from build123d import *

# Parameters (mm, degrees)
BASPROSKE_W        = 16
BASPROSKE_H        = 17
TOOTHCUT_DEPTH     = 29.879058156
TEETHCUTS_COUNT    = 15
TEETHCUTS_ANGLE    = 336
BORSKE_R           = 4
BORE_DEPTH         = 50.0000508
CUT_EXTRUDE1_DEPTH = 5


with BuildPart() as part:
    # BasProSke → Base-Revolve (revolve)
    with BuildSketch(Plane(origin=(0, 0, 0), x_dir=(1, 0, 0), z_dir=(0, 1, 0)), mode=Mode.PRIVATE) as base_revolve_sk:
        with Locations((8, 8.5)):
            Rectangle(BASPROSKE_W, BASPROSKE_H)
    revolve(base_revolve_sk.sketch.rotate(Axis((-10, 0, 0), (1, 0, 0)), 180), axis=Axis((-10, 0, 0), (1, 0, 0)))

    # TooCutSke → ToothCut (cut, through all)
    with BuildSketch(Plane(origin=(0, 0, 0), x_dir=(0, 0, -1), z_dir=(1, 0, 0))):
        with BuildLine():
            ThreePointArc((1.050056448, 12.454813626), (0, 12.499), (-1.050056448, 12.454813626))
            ThreePointArc((-1.050056448, 12.454813626), (-1.638118106, 14.809604533), (-3.110934279, 16.73876737))
            ThreePointArc((-3.110934279, 16.73876737), (0, 17.0254), (3.110934279, 16.73876737))
            ThreePointArc((3.110934279, 16.73876737), (1.638118106, 14.809604533), (1.050056448, 12.454813626))
        make_face()
    toothcut = extrude(amount=TOOTHCUT_DEPTH, mode=Mode.SUBTRACT)

    # TeethCuts: ToothCut ×15 about axis
    teethcuts_axis = Axis((-10, 0, 0), (1, 0, 0))
    for i in range(1, TEETHCUTS_COUNT):
        add(toothcut.rotate(teethcuts_axis, i * TEETHCUTS_ANGLE / (TEETHCUTS_COUNT - 1)), mode=Mode.SUBTRACT)

    # BorSke → Bore (cut, symmetric)
    with BuildSketch(Plane(origin=(0, 0, 0), x_dir=(0, 0, -1), z_dir=(1, 0, 0))):
        with Locations(Location((0, 0, 0), (0, 0, 180))):
            Circle(BORSKE_R)
    extrude(amount=BORE_DEPTH, both=True, mode=Mode.SUBTRACT)

    # Sketch1 → Cut-Extrude1 (cut)
    with BuildSketch(Plane(origin=(16, 0, 0), x_dir=(0, 0, -1), z_dir=(1, 0, 0))):
        Polygon((-3.75277675, 6.5), (-7.505553499, 0), (-3.75277675, -6.5), (3.75277675, -6.5), (7.505553499, 0), (3.75277675, 6.5), align=None)
    extrude(amount=-CUT_EXTRUDE1_DEPTH, mode=Mode.SUBTRACT)


solid = part.part
The listing builds one solid part. Answer for the finished solid, in the listing's coordinates (mm). A direction names the side the tool comes from. Round coordinates to 2 decimals unless told otherwise and drop trailing zeros. Write each loop counter-clockwise with the first axis right and the second up, starting at its lowest first coordinate (ties: lowest second). Pieces come first, ordered by that corner, then holes. Notation, with made-up numbers: (62, 43) - (99, 43) arc R37 cw to (99, 80) - close; hole circle Ø10 at (-9.5, -2). An arc over 180 degrees is marked (long way). Use one line per item in the form item = value. Start each with the question number.
Item 1: Determine the mould class of faces 4 (the cylindrical face through (7.89, -6.24, 10.83)), 5 (the flat face through (0, 3, -4)), 6 (the cylindrical face through (7.888, -14.159, 4.692)) for opening direction Y: +Y half, -Y half, draft (parallel to the pull), parting line (faces both ways), or undercut.
Item 2: A tool of negligible diameter and unlimited length cuts with its end or side. For faces 1 (the cylindrical face through (7.89, 11.41, -5.1)), 2 (the flat face through (13.54, 3.2, -5.66)), 3 (the cylindrical face through (7.9, 11.1, 9.9)), from which of +Z, -Z, +X, -X, +Y, -Y can it reach the whole face along a straight path? Write none if from no direction.
Item 3: Find the intervals of material crossed by line 1 (Y direction, x = 5, z = 0); line 2 (Y direction, x = 2.75, z = -13); line 3 (Z direction, x = 6.5, y = -10), in increasing order. Write a range as [from, to].
Item 4: A cutting plane is placed at C-C (y = -9). Write down the section's boundary in (x, z), plus the area to 3 significant figures.
Item 5: A cutting plane is placed at B-B (z = 14). Write down the section's boundary in (x, y), plus the area to 3 significant figures.
Item 6: Flat-ended cylindrical pins translate along their axes: pin 1 Ø4 at (y, z) = (1, -3) entering from +X; pin 2 Ø3 at (x, z) = (14, -12) entering from -Y; pin 3 Ø1.5 at (x, z) = (12.5, 8.5) entering from +Y. Find the tip coordinate at first contact, or state that the pin passes through.
Item 7: A cutting plane is placed at A-A (z = 0). Write down the section's boundary in (x, y).
The answers:
q1.face_4 = undercut
q1.face_5 = draft
q1.face_6 = -Y half
q2.face_1 = +X, -X
q2.face_2 = +X
q2.face_3 = +Z, +X, -X
q3.line_1 = [-17, -4], [4, 12.5]
q3.line_2 = [-5.9, -2.5], [-0.27, 3.02], [5.65, 8.88]
q3.line_3 = [-12.63, -8.65], [-7.5, 7.5], [8.65, 12.63]
q4.outline = (0, -12.12) - (16, -12.12) - (16, 12.12) - (0, 12.12) - close
q4.area = 388 mm^2
q5.outline = (0, -6) - (16, -6) - (16, -2.87) - (0, -2.87) - close; (0, -0.16) - (16, -0.16) - (16, 3.07) - (0, 3.07) - close; (0, 6.58) - (16, 6.58) - (16, 8.93) - (0, 8.93) - close
q5.area = 139 mm^2
q6.pin_1 = 11
q6.pin_2 = -11.71
q6.pin_3 = 13.89
q7.outline = (0, -17) - (16, -17) - (16, -6.5) - (11, -6.5) - (11, -4) - (0, -4) - close; (0, 4) - (11, 4) - (11, 6.5) - (16, 6.5) - (16, 12.5) - (0, 12.5) - close
